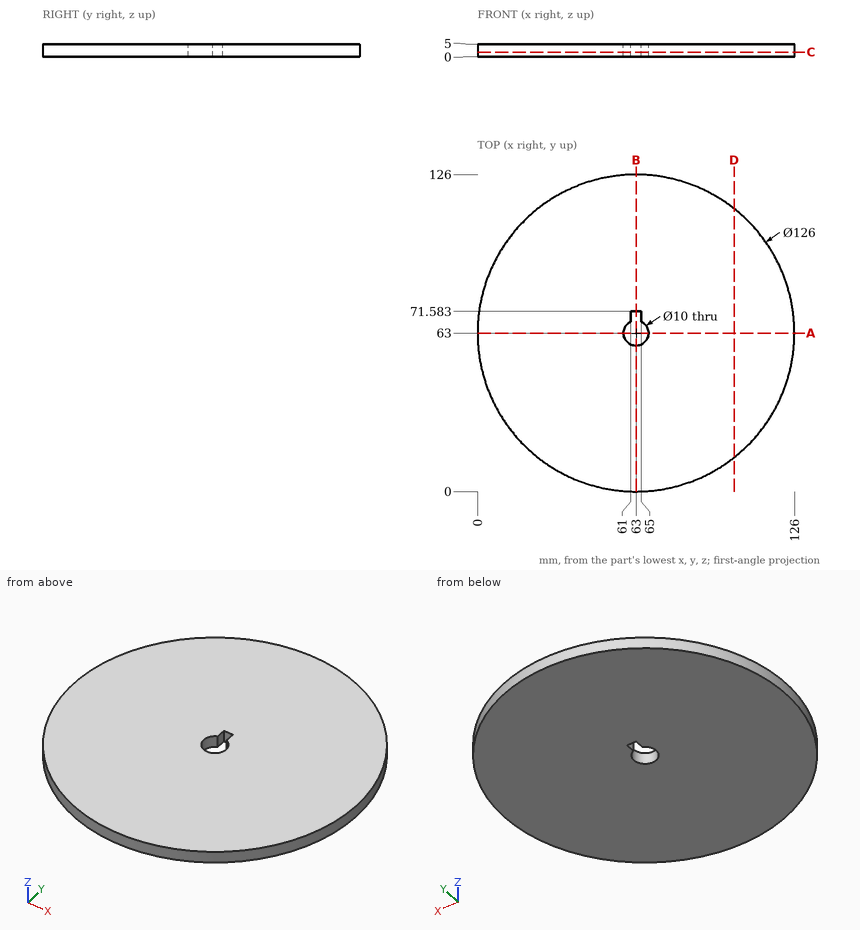
Can you work these out from the drawing? Everything is in mm from the part's minimum corner. Coordinates: 2 decimals unless noted, no trailing zeros. Loops run counter-clockwise (first coordinate to the right, second up) from the corner with the lowest first, then second, coordinate; pieces in that order, holes last. Notation, with made-up numbers: M 68.5,-17.75 L 126.5,-17.75 A9 ccw 126.5,-4.75 Z; hole C 7.5,-23.5 d3. An arc over 180 degrees is marked long. One line per item, written item: value.
1. Imagine slicing it at A-A (y = 63). List the corners of the cut face in (x, z) for me.
Geometry says:
outline: M 0,0 L 58,0 L 58,5 L 0,5 Z; M 68,0 L 126,0 L 126,5 L 68,5 Z
2. Imagine slicing it at D-D (x = 102). List the corners of the cut face in (y, z) for me, and give its area (3 significant figures).
Geometry says:
outline: M 13.52,0 L 112.48,0 L 112.48,5 L 13.52,5 Z
area: 495 mm2
3. Please list where these lines run through material, in increasing order: probe 1 along Y at (x, z) = (63, 2.45); probe 2 along X at (y, z) = (63.5, 2) (1 decimal); probe 3 along Y at (x, z) = (26.5, 2).
Geometry says:
probe 1: y = 0 to 58, 71.58 to 126
probe 2: x = 0 to 58, 68 to 126
probe 3: y = 11.65 to 114.35
4. Imagine slicing it at C-C (z = 1.75). List the corners of the cut face in (x, y) for me, and give its area (3 significant figures).
Geometry says:
outline: C 63,63 d126; hole M 61,67.58 A5 ccw long 65,67.58 L 65,71.58 L 61,71.58 Z
area: 12,400 mm2
5. Will these pins go through, and if not, where does the flat tip stop? pin 1 Ø2 at (y, z) = (74.5, 3) entering from +X; pin 2 Ø3 at (y, z) = (18.5, 2) entering from -X (1 decimal); pin 3 Ø2 at (y, z) = (13.5, 2) entering from +X.
Geometry says:
pin 1: stops at x = 125.12
pin 2: stops at x = 17
pin 3: stops at x = 103.21
6. Imagine slicing it at B-B (x = 63). List the corners of the cut face in (y, z) for me.
Geometry says:
outline: M 0,0 L 58,0 L 58,5 L 0,5 Z; M 71.58,0 L 126,0 L 126,5 L 71.58,5 Z
